from build123d import *

# Parameters (mm, degrees)
SKETCH_1_R      = 5.0225
SKETCH_1_R_2    = 2.05
EXTRUDE_1_DEPTH = 3
FILLET_1_R      = 2
FILLET_2_R      = 1.3
EXTRUDE_START   = -3
SKETCH_3_R      = 5.025
EXTRUDE_2_DEPTH = 3


with BuildPart() as part:
    # 草图1 → 凸台-拉伸1 (new body)
    with BuildSketch(Plane.XY):
        with BuildLine():
            Line((298.545628784, -83.894391363), (298.545628784, -92.841778663))
            Line((298.545628784, -92.841778663), (302.545628784, -92.841778663))
            Line((302.545628784, -92.841778663), (302.545628784, -91.391778663))
            Line((302.545628784, -91.391778663), (305.745628784, -91.391778663))
            Line((305.745628784, -91.391778663), (305.745628784, -92.841778663))
            Line((305.745628784, -92.841778663), (308.945628784, -92.841778663))
            Line((308.945628784, -92.841778663), (308.945628784, -96.941778663))
            Line((308.945628784, -96.941778663), (305.745628784, -96.941778663))
            Line((305.745628784, -96.941778663), (305.745628784, -98.391778663))
            Line((305.745628784, -98.391778663), (302.545628784, -98.391778663))
            Line((302.545628784, -98.391778663), (302.545628784, -96.941778663))
            Line((302.545628784, -96.941778663), (298.545628784, -96.941778663))
            Line((298.545628784, -96.941778663), (298.545628784, -105.894391358))
            Line((298.545628784, -105.894391358), (293.545628784, -105.894391358))
            Line((293.545628784, -105.894391358), (293.545628784, -113.894391358))
            Line((293.545628784, -113.894391358), (298.545628784, -113.894391358))
            Line((298.545628784, -113.894391358), (298.545628784, -122.847004054))
            Line((298.545628784, -122.847004054), (302.545628784, -122.847004054))
            Line((302.545628784, -122.847004054), (302.545628784, -121.397004054))
            Line((302.545628784, -121.397004054), (305.745628784, -121.397004054))
            Line((305.745628784, -121.397004054), (305.745628784, -122.847004054))
            Line((305.745628784, -122.847004054), (308.945628784, -122.847004054))
            Line((308.945628784, -122.847004054), (308.945628784, -126.947004054))
            Line((308.945628784, -126.947004054), (305.745628784, -126.947004054))
            Line((305.745628784, -126.947004054), (305.745628784, -128.397004054))
            Line((305.745628784, -128.397004054), (302.545628784, -128.397004054))
            Line((302.545628784, -128.397004054), (302.545628784, -126.947004054))
            Line((302.545628784, -126.947004054), (298.545628784, -126.947004054))
            Line((298.545628784, -126.947004054), (298.545628784, -140.447004054))
            Line((298.545628784, -140.447004054), (324.188862368, -140.447004054))
            Line((324.188862368, -140.447004054), (376.358604426, -71.946984141))
            Line((376.358604426, -71.946984141), (376.358604426, 4.396201153))
            ThreePointArc((376.358604426, 4.396201153), (348.536987634, 32.217817945), (320.715370843, 4.396201153))
            Line((320.715370843, 4.396201153), (307.936987634, -35.096984141))
            Line((307.936987634, -35.096984141), (298.545628784, -35.096984141))
            Line((298.545628784, -35.096984141), (298.545628784, -45.889165972))
            Line((298.545628784, -45.889165972), (293.545628784, -45.889165972))
            Line((293.545628784, -45.889165972), (293.545628784, -53.889165972))
            Line((293.545628784, -53.889165972), (298.545628784, -53.889165972))
            Line((298.545628784, -53.889165972), (298.545628784, -62.841778668))
            Line((298.545628784, -62.841778668), (302.545628784, -62.841778668))
            Line((302.545628784, -62.841778668), (302.545628784, -61.391778668))
            Line((302.545628784, -61.391778668), (305.745628784, -61.391778668))
            Line((305.745628784, -61.391778668), (305.745628784, -62.841778668))
            Line((305.745628784, -62.841778668), (308.945628784, -62.841778668))
            Line((308.945628784, -62.841778668), (308.945628784, -66.941778668))
            Line((308.945628784, -66.941778668), (305.745628784, -66.941778668))
            Line((305.745628784, -66.941778668), (305.745628784, -68.391778668))
            Line((305.745628784, -68.391778668), (302.545628784, -68.391778668))
            Line((302.545628784, -68.391778668), (302.545628784, -66.941778668))
            Line((302.545628784, -66.941778668), (298.545628784, -66.941778668))
            Line((298.545628784, -66.941778668), (298.545628784, -75.894391363))
            Line((298.545628784, -75.894391363), (293.545628784, -75.894391363))
            Line((293.545628784, -75.894391363), (293.545628784, -83.894391363))
            Line((293.545628784, -83.894391363), (298.545628784, -83.894391363))
        make_face()
        with Locations((348.536987634, 4.396201153)):
            Circle(SKETCH_1_R, mode=Mode.SUBTRACT)
        with Locations((320.545628784, -134.447004054)):
            Circle(SKETCH_1_R_2, mode=Mode.SUBTRACT)
        with Locations((370.358604426, -65.946984141)):
            Circle(SKETCH_1_R_2, mode=Mode.SUBTRACT)
        with Locations((313.936987634, -41.346984141)):
            Circle(SKETCH_1_R_2, mode=Mode.SUBTRACT)
        Polygon((354.947285032, -70.136765586), (328.579617375, -106.396108383), (325.08144343, -57.115165973), align=None, mode=Mode.SUBTRACT)
        Polygon((329.571126451, -37.254352656), (354.337315751, -48.052488042), (344.758747766, -17.175445836), align=None, mode=Mode.SUBTRACT)
    extrude(amount=EXTRUDE_1_DEPTH)

    # 圆角1
    fillet_1_edges = [part.edges().sort_by_distance(p)[0] for p in [
        (354.947285032, -70.136765586, 1.5),
        (325.08144343, -57.115165973, 1.5),
        (328.579617375, -106.396108383, 1.5),
        (344.758747766, -17.175445836, 1.5),
        (329.571126451, -37.254352656, 1.5),
        (354.337315751, -48.052488042, 1.5),
    ]]
    fillet(fillet_1_edges, radius=FILLET_1_R)

    # 圆角2
    fillet_2_edges = [part.edges().sort_by_distance(p)[0] for p in [
        (293.545628784, -113.894391358, 1.5),
        (293.545628784, -105.894391358, 1.5),
        (293.545628784, -83.894391363, 1.5),
        (293.545628784, -75.894391363, 1.5),
        (293.545628784, -53.889165972, 1.5),
        (293.545628784, -45.889165972, 1.5),
    ]]
    fillet(fillet_2_edges, radius=FILLET_2_R)

    # 草图3 → 凸台-拉伸2 (add)
    with BuildSketch(Plane(origin=(0, 0, 0), x_dir=(-1, 0, 0), z_dir=(0, 0, -1)).offset(EXTRUDE_START)):
        with BuildLine():
            Line((-348.536987634, 28.396201153), (-396.833278949, 30.337153408))
            ThreePointArc((-396.833278949, 30.337153408), (-409.833278949, 17.337153408), (-396.833278949, 4.337153408))
            Line((-396.833278949, 4.337153408), (-348.536987634, -19.603798847))
            Line((-348.536987634, -19.603798847), (-372.536987634, 4.396201153))
            Line((-372.536987634, 4.396201153), (-348.536987634, 28.396201153))
        make_face()
        with Locations((-396.833278949, 17.337153408)):
            Circle(SKETCH_3_R, mode=Mode.SUBTRACT)
    extrude(amount=EXTRUDE_2_DEPTH)


solid = part.part
Input: part model. Units: mm. Frame: model coordinates. A direction names the side the tool comes from. Coordinates: 2 decimals unless noted, no trailing zeros. Loops run counter-clockwise (first coordinate to the right, second up) from the corner with the lowest first, then second, coordinate; pieces in that order, holes last. Notation, with made-up numbers: (65.5, -35.5) -> (70.5, -35.5) arc R7 ccw to (70.5, -22.5) -> close; hole circle Ø2 at (44.25, 74). An arc over 180 degrees is marked (long way). Write item = value, one per line. Start each with the question number.
Item 1: Cut plane D-D, the plane z = 1.4. Count the separate pieces of the cut face and the enclosed holes in it, plus the area to 3 significant figures.
Item 2: Material intervals for line 1 (Y direction, x = 307.5, z = 0.8); line 2 (Y direction, x = 298.5, z = 0.5); line 3 (Y direction, x = 337, z = 2.75), sorted ascending.
Item 3: Cut plane B-B, the plane y = -50. Return loops of the section in (x, z).
Item 4: Mould query, pull axis X, two halves, no side actions, for faces 3 (the face through (368.31, -65.86, 1.48)), 4 (the face through (386.739, -0.667, 1.521)), 5 (the face through (314.416, -15.074, 1.479)). Classes: pulls with the +X half, pulls with the -X half, needs draft (parallel to the pull), parting line crosses it, or undercut.
Item 5: First-contact query: P1, Ø1.6, axis at y = -92.5, z = 1, coming from the +X side; P2, Ø0.7, axis at y = -128, z = 1, coming from the +X side; P3, Ø8, axis at x = 380, y = -47, coming from the +Z side; P4, Ø2, axis at x = 343.5, y = -21.5, coming from the +Z side. Flat tips, straight axial feed; report the tip coordinate or a pass-through.
Item 6: Cut plane A-A, the plane y = 20. Return loops of the section in (x, z).
Item 7: Cut plane C-C, the plane x = 379.5. Return loops of the section in (y, z).
Item 8: Reachability of faces 1 (the face through (349.909, -106.676, 1.479)), 2 (the face through (336.8, -27.7, 1.5)) from +Z, -Z, +X, -X, +Y, -Y: full face, straight path, thin tool, end or side. Return the list, or none.
Ans:
q1.separate_pieces = 1
q1.enclosed_holes = 7
q1.area = 9,820 mm²
q2.line_1 = -140.45 to -126.95, -122.85 to -96.94, -92.84 to -66.94, -62.84 to -35.1
q2.line_2 = -113.89 to -105.89, -83.89 to -75.89, -53.89 to -45.89
q2.line_3 = -123.63 to -94.82, -62.31 to -40.49, -27.43 to 29.71
q3.outline = (293.55, 0) -> (376.36, 0) -> (376.36, 3) -> (293.55, 3) -> close
q4.face_3 = undercut
q4.face_4 = pulls with the +X half
q4.face_5 = pulls with the -X half
q5.P1 = 361.31
q5.P2 = 333.94
q5.P3 = 3
q5.P4 = through
q6.outline = (325.5, 0) -> (392.57, 0) -> (392.57, 3) -> (325.5, 3) -> close; (401.09, 0) -> (409.56, 0) -> (409.56, 3) -> (401.09, 3) -> close
q7.outline = (-4.26, 0) -> (29.64, 0) -> (29.64, 3) -> (-4.26, 3) -> close
q8.face_1 = +Z, -Z, +X, -Y
q8.face_2 = +Z, -Z
